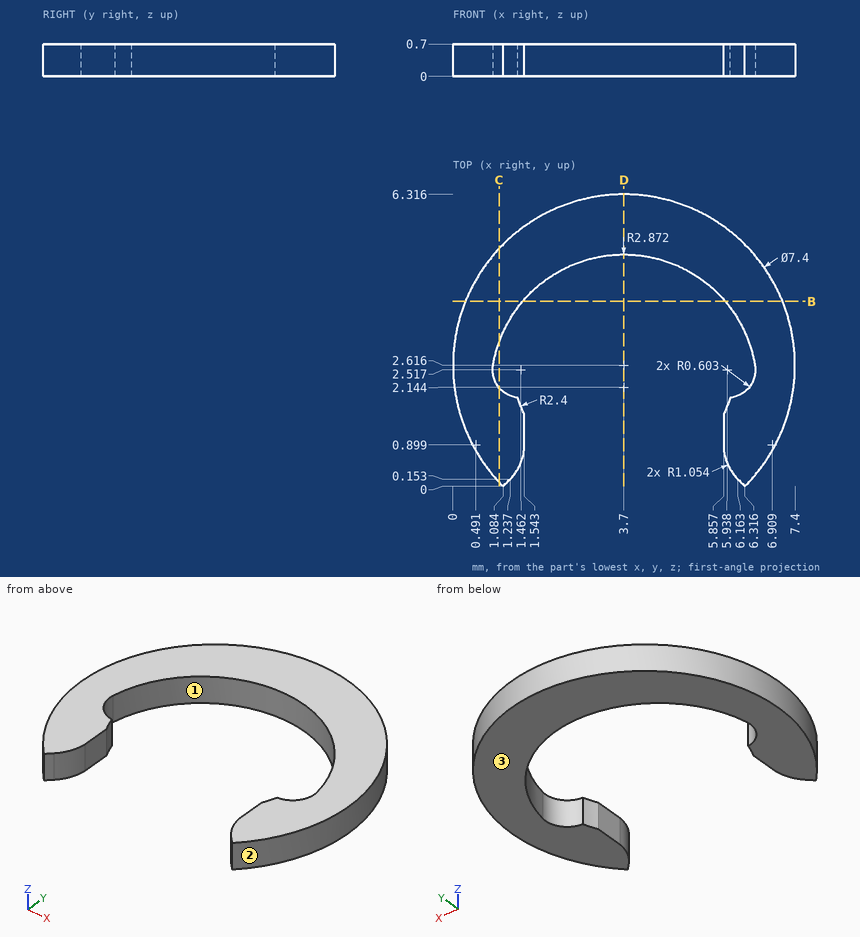
The drawing under review shows one solid part. Ordinate dimensions are in mm from its lowest x, y, z. Give positions to 0.01 mm unless a question says otherwise; leave off trailing zeros. Order: outer loops, then holes, each group sorted by start corner. A loop starts at its lowest first (then second) coordinate and runs counter-clockwise, first axis right, second up. Notation, with made-up numbers: M 7.5,71 L 62.5,71 A37 cw 62.5,109 Z; hole C 41.5,53 d5. An arc over 180 degrees is marked long. Answer in a Markdown table with one row per item. Add a question column.
1. Add section C-C on x = 1. State the section outline as (y, z) points (1 decimal).
2. Add section B-B on y = 4. State the section outline as (x, z) points.
3. To check wall thickness, follow line 1 along X through (y, z) = (2.5, 0.55); line 2 along X through (y, z) = (0.5, 0.6) (1 decimal); line 3 along Y through (x, z) = (3.75, 0.15) (1 decimal). State the ranges of each line that lie inside material, in increasing order.
4. Add section D-D on x = 3.7. State the section outline as (y, z) points.
5. Mouldability with a two-part tool opening along Y and no side actions: class the marked faces 1, 2 and 3 as released by +Y, released by -Y, zero draft, split by the parting line, or undercut.
The answers:
| question | item | result |
|---|---|---|
| 1 | outline | M 0.1,0 L 2.1,0 L 2.1,0.7 L 0.1,0.7 Z; M 3.1,0 L 5.1,0 L 5.1,0.7 L 3.1,0.7 Z |
| 2 | outline | M 0.27,0 L 1.51,0 L 1.51,0.7 L 0.27,0.7 Z; M 5.89,0 L 7.13,0 L 7.13,0.7 L 5.89,0.7 Z |
| 3 | line 1 | 0 to 0.86, 6.54 to 7.4 |
| 3 | line 2 | 0.7 to 1.5, 5.9 to 6.7 |
| 3 | line 3 | 5 to 6.3 |
| 4 | outline | M 5.02,0 L 6.32,0 L 6.32,0.7 L 5.02,0.7 Z |
| 5 | face 1 | undercut |
| 5 | face 2 | split by the parting line |
| 5 | face 3 | zero draft |
